from build123d import *

# Parameters (mm, degrees)
F0_R     = 6.35
F1_DEPTH = 3.175


with BuildPart() as f1:
    # F0 (on Right) → F1 (new body, symmetric)
    with BuildSketch(Plane.YZ):
        with BuildLine():
            Line((15.875, -300), (15.875, 0))
            ThreePointArc((15.875, 0), (0, 15.875), (-15.875, 0))
            Line((-15.875, 0), (-15.875, -300))
            ThreePointArc((-15.875, -300), (0, -315.875), (15.875, -300))
        make_face()
        with Locations((0, -300)):
            Circle(F0_R, mode=Mode.SUBTRACT)
        Circle(F0_R, mode=Mode.SUBTRACT)
    extrude(amount=F1_DEPTH, both=True)


solid = f1.part
Design review of the part built by this model. Coordinates are the model's own, in mm. Coordinates: 2 decimals unless noted, no trailing zeros. Order: outer loops, then holes, each group sorted by start corner. A loop starts at its lowest first (then second) coordinate and runs counter-clockwise, first axis right, second up.
Item 1: Take a section at A-A, the plane y = 0. Write out the cut boundary in (x, z) (3 decimals), then the cut area to 3 significant figures.
Item 2: Take a section at B-B, the plane x = -0.5. Write out the cut boundary in (y, z) (3 decimals), then the cut area to 3 significant figures.
Item 3: For line 1 (Z direction, x = -1, y = 0) (3 decimals); line 2 (Y direction, x = 0, z = -300) (3 decimals); line 3 (Z direction, x = 0.25, y = -4), list the stretches that pass through material, from the lowest coordinate up.
Item 4: The part is to be moulded in two halves that separate along Z. For faces 1 (the cylindrical face through (-0.04, -1.38, -6.2)), 2 (the flat face through (-3.175, 0, -148)), 3 (the cylindrical face through (0.04, -0.35, -315.87)), say which applies: pulls with the +Z half, pulls with the -Z half, needs draft (parallel to the pull), parting line crosses it, or undercut.
Item 5: For pin 1 Ø1 at (x, y) = (-1.5, 3.5) entering from +Z; pin 2 Ø11.5 at (y, z) = (0, 0) entering from +X, all flat-tipped, find the tip position at first contact; note any pin that passes through.
The answers:
1. outline: (-3.175, -315.875) - (3.175, -315.875) - (3.175, -306.35) - (-3.175, -306.35) - close; (-3.175, -293.65) - (3.175, -293.65) - (3.175, -6.35) - (-3.175, -6.35) - close; (-3.175, 6.35) - (3.175, 6.35) - (3.175, 15.875) - (-3.175, 15.875) - close
1. area: 1,950 mm2
2. outline: (-15.875, -300) arc R15.875 ccw to (15.875, -300) - (15.875, 0) arc R15.875 ccw to (-15.875, 0) - close; hole circle Ø12.7 at (0, -300); hole circle Ø12.7 at (0, 0)
2. area: 10,100 mm2
3. line 1: z = -315.875 to -306.35, -293.65 to -6.35, 6.35 to 15.875
3. line 2: y = -15.875 to -6.35, 6.35 to 15.875
3. line 3: z = -315.36 to -304.93, -295.07 to -4.93, 4.93 to 15.36
4. face 1: undercut
4. face 2: needs draft
4. face 3: pulls with the -Z half
5. pin 1: stops at z = 15.59
5. pin 2: passes through
